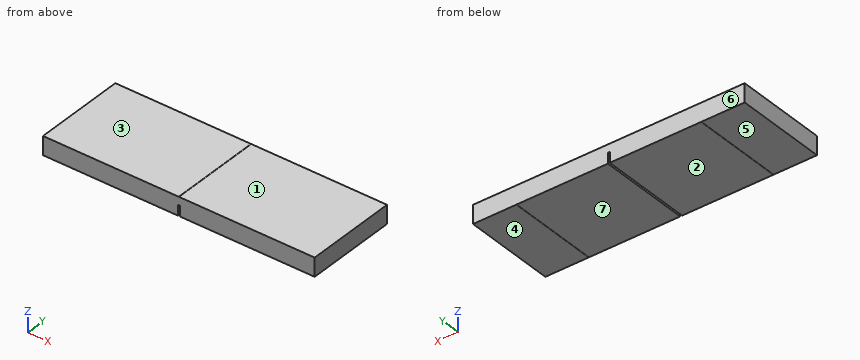
```python
from build123d import *

# Parameters (mm, degrees)
F0_W     = 7.35295
F0_H     = 1
F1_DEPTH = 5
F2_W     = 0.051922
F2_H     = 0.562747
F3_DEPTH = 5.001
F4_W     = 0.005
F4_H     = 5
F5_DEPTH = 0.01
F6_W     = 0.005
F6_H     = 5
F7_DEPTH = 0.01


with BuildPart() as f1:
    # F0 (on Front) → F1 (new body)
    with BuildSketch(Plane.XZ):
        with Locations((3.676475, 0)):
            Rectangle(F0_W, F0_H)
        with Locations((-3.676475, 0)):
            Rectangle(F0_W, F0_H)
    extrude(amount=F1_DEPTH)

    # F2 (on face) → F3 (cut, through all)
    with BuildSketch(Plane.XZ.offset(5)):
        with Locations((-0.025961, -0.218627)):
            Rectangle(F2_W, F2_H)
        with Locations((0.025961, -0.218627)):
            Rectangle(F2_W, F2_H)
    extrude(amount=-F3_DEPTH, mode=Mode.SUBTRACT)

    # F4 (on face) → F5 (join)
    with BuildSketch(Plane.XY.offset(0.5)):
        with Locations((-0.0025, -2.5)):
            Rectangle(F4_W, F4_H)
        with Locations((0.0025, -2.5)):
            Rectangle(F4_W, F4_H)
    extrude(amount=F5_DEPTH)

    # F6 (on face) → F7 (join)
    with BuildSketch(Plane(origin=(0, 0, -0.5), x_dir=(1, 0, 0), z_dir=(0, 0, -1))):
        with Locations((-4.9975, 2.5)):
            Rectangle(F6_W, F6_H)
        with Locations((-5.0025, 2.5)):
            Rectangle(F6_W, F6_H)
        with Locations((5.0025, 2.5)):
            Rectangle(F6_W, F6_H)
        with Locations((4.9975, 2.5)):
            Rectangle(F6_W, F6_H)
    extrude(amount=F7_DEPTH)


solid = f1.part
```
The listing builds one solid part. Answer for the finished solid, in the listing's coordinates (mm). Face numbers are marked on the shaded views. A direction names the side the tool comes from. Round coordinates to 2 decimals unless told otherwise and drop trailing zeros. Order: outer loops, then holes, each group sorted by start corner. A loop starts at its lowest first (then second) coordinate and runs counter-clockwise, first axis right, second up. Notation, with made-up numbers: (61, 19) - (115, 19) arc R23 cw to (115, 50) - close; hole circle Ø2 at (16, -35.5). An arc over 180 degrees is marked (long way). Put each result on its own line as item: value. Start each with the question number.
(1) Find section B-B (x = 6). Give the vertices of the cut face in (y, z).
(2) Determine the mould class of the marked faces 6 and 7 for opening direction X: released by +X, released by -X, zero draft, split by the parting line, or undercut.
(3) A straight line is drawn through the part: probe 1 along Z at (x, y) = (-0.75, -1.6). Find the intervals that lie inside material, in ascending order. Write a range as from..to.
(4) Find section A-A (y = -2.75). Give the vertices of the cut face in (x, z) (3 decimals).
(5) For the marked faces 1, 2, 3, 4 and 5, determine the directions among +Z, -Z, +X, -X, +Y, -Y from which every point of the face is accessible in a straight line to the end or side of a thin tool.
(6) Given P1, Ø1.5, axis at x = -3, y = -3, coming from the +Z side; P2, Ø1, axis at x = -0.5, y = -1.5, coming from the -Z side, each flat-ended and moving along its own axis, determine where each tip first touches the part or whether it passes through.
Reply:
1. outline: (-5, -0.5) - (0, -0.5) - (0, 0.5) - (-5, 0.5) - close
2. face 6: zero draft
2. face 7: undercut
3. probe 1: -0.5..0.5
4. outline: (-7.353, -0.5) - (-5.005, -0.5) - (-5.005, -0.51) - (-4.995, -0.51) - (-4.995, -0.5) - (-0.052, -0.5) - (-0.052, 0.063) - (0.052, 0.063) - (0.052, -0.5) - (4.995, -0.5) - (4.995, -0.51) - (5.005, -0.51) - (5.005, -0.5) - (7.353, -0.5) - (7.353, 0.5) - (0.005, 0.5) - (0.005, 0.51) - (-0.005, 0.51) - (-0.005, 0.5) - (-7.353, 0.5) - close
5. face 1: +Z, +X, +Y, -Y
5. face 2: -Z, +Y, -Y
5. face 3: +Z, -X, +Y, -Y
5. face 4: -Z, +X, +Y, -Y
5. face 5: -Z, -X, +Y, -Y
6. P1: z = 0.5
6. P2: z = -0.5
